Verification items for this drawing (mm, ordinates from the low corner). Coordinates: 2 decimals unless noted, no trailing zeros. Write each loop counter-clockwise with the first axis right and the second up, starting at its lowest first coordinate (ties: lowest second). Pieces come first, ordered by that corner, then holes.
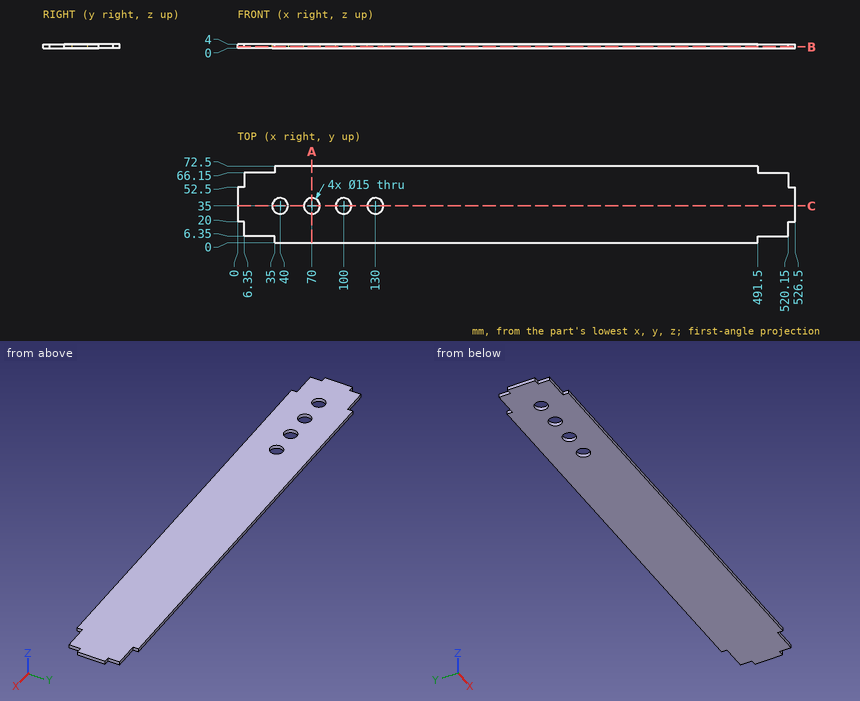
1. Sectioned sample at A-A, the plane x = 70. Record the boundary of the cut face in (y, z), and give its area (3 significant figures).
Computed values:
outline: (0, 0) - (27.5, 0) - (27.5, 4) - (0, 4) - close; (42.5, 0) - (72.5, 0) - (72.5, 4) - (42.5, 4) - close
area: 230 mm2
2. Sectioned sample at B-B, the plane z = 1.2. Record the boundary of the cut face in (x, y), and give its area (3 significant figures).
Computed values:
outline: (0, 20) - (6.35, 20) - (6.35, 6.35) - (35, 6.35) - (35, 0) - (491.5, 0) - (491.5, 6.35) - (520.15, 6.35) - (520.15, 20) - (526.5, 20) - (526.5, 52.5) - (520.15, 52.5) - (520.15, 66.15) - (491.5, 66.15) - (491.5, 72.5) - (35, 72.5) - (35, 66.15) - (6.35, 66.15) - (6.35, 52.5) - (0, 52.5) - close; hole circle Ø15 at (40, 35); hole circle Ø15 at (70, 35); hole circle Ø15 at (100, 35); hole circle Ø15 at (130, 35)
area: 36,200 mm2
3. Thickness scan on line 1 along Y through (x, z) = (71, 0.6); line 2 along Y through (x, z) = (70, 1); line 3 along X through (y, z) = (58.5, 1.8). Record the ranges inside material, lowest first.
Computed values:
line 1: y = 0 to 27.57, 42.43 to 72.5
line 2: y = 0 to 27.5, 42.5 to 72.5
line 3: x = 6.35 to 520.15
4. Sectioned sample at C-C, the plane y = 35. Record the boundary of the cut face in (x, z).
Computed values:
outline: (0, 0) - (32.5, 0) - (32.5, 4) - (0, 4) - close; (47.5, 0) - (62.5, 0) - (62.5, 4) - (47.5, 4) - close; (77.5, 0) - (92.5, 0) - (92.5, 4) - (77.5, 4) - close; (107.5, 0) - (122.5, 0) - (122.5, 4) - (107.5, 4) - close; (137.5, 0) - (526.5, 0) - (526.5, 4) - (137.5, 4) - close
5. Gauge pin test, flat ends, axial feed: pin 1 Ø1.2 at (x, z) = (507, 2.5) entering from +Y; pin 2 Ø1 at (y, z) = (64, 0.5) entering from +X; pin 3 Ø2 at (x, z) = (2.5, 1.5) entering from +Y. Record the tip position at first contact, or that the pin passes through.
Computed values:
pin 1: stops at y = 66.15
pin 2: stops at x = 520.15
pin 3: stops at y = 52.5
